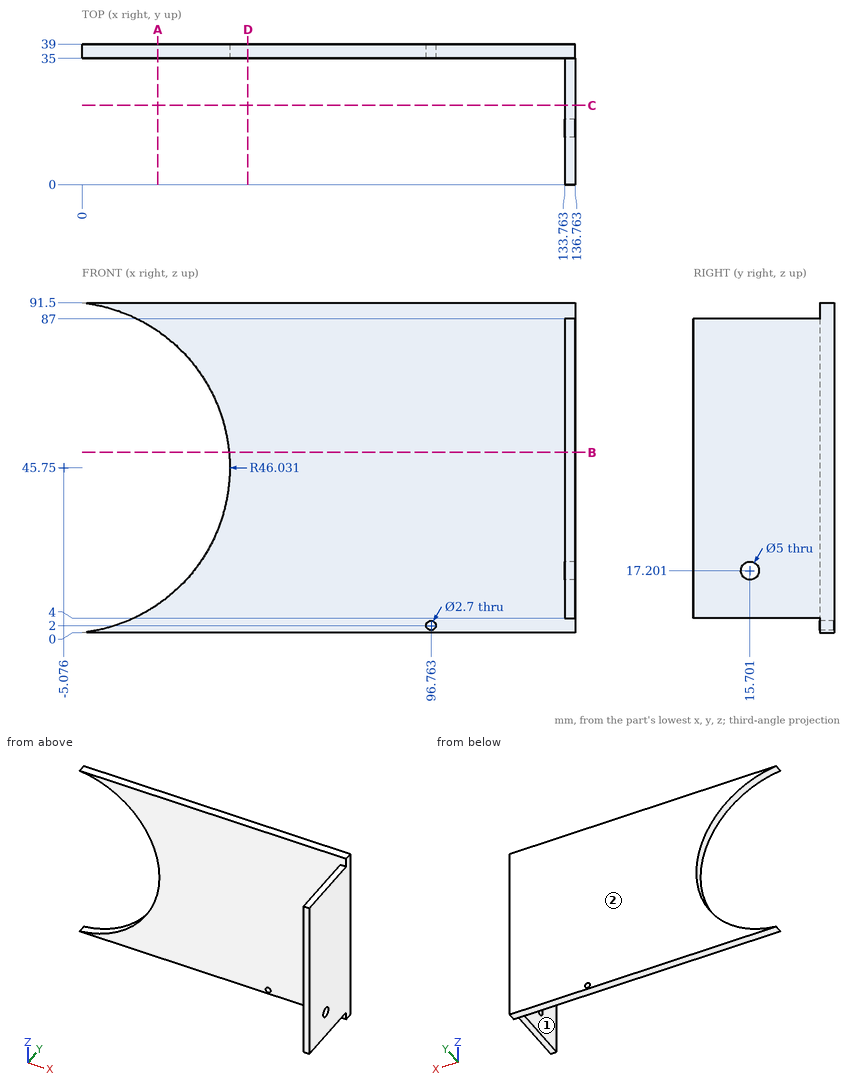
Source: three-view drawing plus pictorial views. Frame: mm from the lowest corner of the part. A direction names the side the tool comes from. Give positions to 0.01 mm unless a question says otherwise; leave off trailing zeros. Order: outer loops, then holes, each group sorted by start corner. A loop starts at its lowest first (then second) coordinate and runs counter-clockwise, first axis right, second up. Notation, with made-up numbers: M 38,60 L 93,60 A23 cw 93,87 Z; hole C -16.75,66.5 d8. An arc over 180 degrees is marked long. Return JSON: item names as keys, results as strings.
1) Access query for the marked faces 1 and 2. Directions: +Z, -Z, +X, -X, +Y, -Y. A direction counts if a zero-diameter tool reaches every point of the face in a straight line with its end or side. Return the directions, or none.
Taken from the geometry:
{"face 1": "+Z, -Z, -X, -Y", "face 2": "+Z, -Z, +X, -X, +Y"}
2) Contact query for flat-ended pins moving along their axis: pin 1 (10 mm diameter, centred on x = 85, z = 29.5, fed in from -Y); pin 2 (1.5 mm diameter, centred on x = 135, y = 19.5, fed in from +Z); pin 3 (6 mm diameter, centred on y = 31.5, z = 56, fed in from -X); pin 4 (10 mm diameter, centred on x = 30, z = 61, fed in from +Y) (3 decimals). Output: stop coordinate, or through.
Taken from the geometry:
{"pin 1": "stops at y = 35", "pin 2": "stops at z = 87", "pin 3": "stops at x = 133.76", "pin 4": "passes through"}
3) Line query: L1, parallel to Y at x = 43, z = 77.5; L2, parallel to X at y = 4.5, z = 47.5; L3, parallel to X at y = 36, z = 9 (1 decimal). Output: solid intervals per line, ascending. Write a range as [from, to].
Taken from the geometry:
{"L1": "y = [35, 39]", "L2": "x = [133.76, 136.76]", "L3": "x = [22.6, 136.8]"}
4) Section query C-C on y = 22. Output: boundary loops of the cut face in (x, z).
Taken from the geometry:
{"outline": "M 133.76,4 L 136.76,4 L 136.76,87 L 133.76,87 Z"}
5) Section query D-D on x = 46. Output: boundary loops of the cut face in (y, z).
Taken from the geometry:
{"outline": "M 35,0 L 39,0 L 39,91.5 L 35,91.5 Z"}
6) Section query A-A on x = 21. Output: boundary loops of the cut face in (y, z).
Taken from the geometry:
{"outline": "M 35,0 L 39,0 L 39,7.82 L 35,7.82 Z; M 35,83.68 L 39,83.68 L 39,91.5 L 35,91.5 Z"}
7) Section query B-B on z = 50. Output: boundary loops of the cut face in (x, y).
Taken from the geometry:
{"outline": "M 40.76,35 L 133.76,35 L 133.76,0 L 136.76,0 L 136.76,39 L 40.76,39 Z"}
